Model file for the job. Use its own axes, mm. A direction names the side the tool comes from. Coordinates: 2 decimals unless noted, no trailing zeros. Order: outer loops, then holes, each group sorted by start corner. A loop starts at its lowest first (then second) coordinate and runs counter-clockwise, first axis right, second up. Notation, with made-up numbers: (9, -0.5) -> (40, -0.5) arc R19 ccw to (40, 3.5) -> close; hole circle Ø11 at (64, 75). An arc over 180 degrees is marked (long way). Return JSON: item names as keys, results as strings. Group by question number.
1) Cut at C-C (y = 73.5). Write the cut outline in (x, z).
2) Cut at B-B (z = -26.5). Write the cut outline in (x, y), and give its area (3 significant figures).
3) Probe line 1 (Y direction, x = 41.75, z = -55); line 2 (X direction, y = 2.55, z = 4); line 3 (X direction, y = 2.1, z = -43). List the from-to ranges inside material, lowest first.
4) Cut at A-A (z = -55). State how many separate pieces and enclosed holes the cut face has, and give its area (3 significant figures).
5) Flat gauge pins, fed straight in: pin 1 (8 mm diameter, centred on x = 38.5, y = 87.5, fed in from +Z); pin 2 (4 mm diameter, centred on x = 33, z = -80.5, fed in from -Y); pin 3 (4 mm diameter, centred on y = 28, z = -54.5, fed in from -X). Where does each tip first touch, or does it go through?
6) Which spindle directions (+Z, -Z, +X, -X, +Y, -Y) get a long thin tool onto all of the face, cutting with end or side? Do faces 1 (the cylindrical face through (38.19, 2.96, -41.45)), 2 (the flat face through (38, 126, -30)), 3 (the flat face through (34.97, 41.13, -55.07)), 4 (the flat face through (38, 121, -83)), 5 (the flat face through (38, 71, 22)). Say none if no direction does.
7) Pull direction Y, two halves, no side cores. Call faces 6 (the flat face through (28, 49, 10)), 7 (the flat face through (13.7, 39.5, -5.1)), 8 (the flat face through (6.375, 17.042, -55.07)): +Y half, -Y half, draft (parallel to the pull), parting line (faces both ways), or undercut.
from build123d import *

# Parameters (mm, degrees)
SKETCH_1_W          = 35
SKETCH_1_H          = 60
SKETCH_1_W_2        = 8
EXTRUDE_1_DEPTH     = 6
HOLE_WIZARD_1_D     = 3.5
FILLET_1_R          = 3
SKETCH_5_W          = 10
SKETCH_5_H          = 10
EXTRUDE_2_DEPTH     = 120
SKETCH_10_W         = 10
SKETCH_10_H         = 60
EXTRUDE_5_DEPTH     = 10
HOLE_WIZARD_2_D     = 3.5
HOLE_WIZARD_3_D     = 6
HOLE_WIZARD_3_DEPTH = 4
EXTRUDE_6_DEPTH     = 10
SKETCH_18_W         = 35
SKETCH_18_H         = 15
EXTRUDE_7_DEPTH     = 10
HOLE_WIZARD_4_D     = 4
FILLET_2_R          = 10
FILLET_3_R          = 3
SKETCH_21_W         = 10
SKETCH_21_H         = 10
EXTRUDE_8_DEPTH     = 6
HOLE_WIZARD_5_D     = 4
SKETCH_25_W         = 10
SKETCH_25_H         = 10
EXTRUDE_9_DEPTH     = 10
SKETCH_28_W         = 4
SKETCH_28_H         = 8
CUT_EXTRUDE_1_DEPTH = 172.37677789
CUT_EXTRUDE_2_DEPTH = 172.37677789


with BuildPart() as part:
    # 草图1 → 凸台-拉伸1 (new body)
    with BuildSketch(Plane(origin=(0, 0, 0), x_dir=(1, 0, 0), z_dir=(0, 1, 0))):
        Polygon((18, 68), (18, 60), (35, 60), (43, 60), (43, 68), align=None)
        with Locations((17.5, 30)):
            Rectangle(SKETCH_1_W, SKETCH_1_H)
        with Locations((39, 30)):
            Rectangle(SKETCH_1_W_2, SKETCH_1_H)
        Polygon((35, 0), (18, 0), (18, -8), (43, -8), (43, 0), align=None)
    extrude(amount=EXTRUDE_1_DEPTH)

    # 孔1 (through all)
    with Locations(Plane(origin=(0, 6, 0), x_dir=(1, 0, 0), z_dir=(0, 1, 0))):
        with Locations((24, 64), (39, 43), (39, 17), (24, -4)):
            Hole(HOLE_WIZARD_1_D / 2)

    # 圆角1
    fillet_1_edges = [part.edges().sort_by_distance(p)[0] for p in [
        (18, 3, 8),
        (18, 3, 0),
        (18, 3, -68),
        (43, 3, -68),
        (43, 3, 8),
    ]]
    fillet(fillet_1_edges, radius=FILLET_1_R)

    # 草图5 → 凸台-拉伸2 (add)
    with BuildSketch(Plane(origin=(0, 6, 0), x_dir=(1, 0, 0), z_dir=(0, 1, 0))):
        with Locations((38, 55)):
            Rectangle(SKETCH_5_W, SKETCH_5_H)
        with Locations((38, 5)):
            Rectangle(SKETCH_5_W, SKETCH_5_H)
    extrude(amount=EXTRUDE_2_DEPTH)

    # 草图10 → 凸台-拉伸5 (add)
    with BuildSketch(Plane(origin=(0, 126, 0), x_dir=(1, 0, 0), z_dir=(0, 1, 0))):
        with Locations((38, 30)):
            Rectangle(SKETCH_10_W, SKETCH_10_H)
    extrude(amount=EXTRUDE_5_DEPTH)

    # 孔2 (through all)
    with Locations(Plane(origin=(43, 0, 0), x_dir=(0, 0, -1), z_dir=(1, 0, 0))):
        with Locations((5, 131), (55, 131), (55, 80), (5, 80)):
            Hole(HOLE_WIZARD_2_D / 2)

    # 孔3
    with Locations(Plane(origin=(43, 0, 0), x_dir=(0, 0, -1), z_dir=(1, 0, 0))):
        with Locations((5, 131), (5, 80), (55, 80), (55, 131)):
            Hole(HOLE_WIZARD_3_D / 2, depth=HOLE_WIZARD_3_DEPTH)

    # 草图16 → 凸台-拉伸6 (add)
    with BuildSketch(Plane(origin=(0, 0, -60), x_dir=(-1, 0, 0), z_dir=(0, 0, -1))):
        Polygon((-33, 51.15767665), (-6.92820323, 6), (0, 6), (-33, 63.15767665), align=None)
    extrude_6 = extrude(amount=-EXTRUDE_6_DEPTH)

    # 镜向1: 凸台-拉伸6 across plane
    add(extrude_6.mirror(Plane.XY.offset(-30)))

    # 草图18 → 凸台-拉伸7 (add)
    with BuildSketch(Plane.ZY.offset(-33)):
        with Locations((-77.5, 128.5)):
            Rectangle(SKETCH_18_W, SKETCH_18_H)
        with Locations((17.5, 128.5)):
            Rectangle(SKETCH_18_W, SKETCH_18_H)
        with Locations((-77.5, 63.5)):
            Rectangle(SKETCH_18_W, SKETCH_18_H)
        with Locations((17.5, 63.5)):
            Rectangle(SKETCH_18_W, SKETCH_18_H)
    extrude(amount=-EXTRUDE_7_DEPTH)

    # 孔4 (through all)
    with Locations(Plane.ZY.offset(-33)):
        with Locations((-87.5, 129), (27.5, 129), (27.5, 63), (-87.5, 63)):
            Hole(HOLE_WIZARD_4_D / 2)

    # 圆角2
    fillet_2_edges = [part.edges().sort_by_distance(p)[0] for p in [
        (38, 121, -60),
        (38, 121, 0),
        (38, 71, -60),
        (38, 71, 0),
    ]]
    fillet(fillet_2_edges, radius=FILLET_2_R)

    # 圆角3
    fillet_3_edges = [part.edges().sort_by_distance(p)[0] for p in [
        (18, 3, -60),
    ]]
    fillet(fillet_3_edges, radius=FILLET_3_R)

    # 草图21 → 凸台-拉伸8 (add)
    with BuildSketch(Plane(origin=(-2.598076211, 1.5, 0), x_dir=(0, 0, 1), z_dir=(-0.8660254037844363, 0.5000000000000042, 0))):
        Polygon((-60, 51.059600438), (-70, 51.059600438), (-60, 41.059600438), align=None)
        with Locations((-65, 56.059600438)):
            Rectangle(SKETCH_21_W, SKETCH_21_H)
        with Locations((5, 56.059600438)):
            Rectangle(SKETCH_21_W, SKETCH_21_H)
        Polygon((0, 51.059600438), (10, 51.059600438), (0, 41.059600438), align=None)
    extrude(amount=-EXTRUDE_8_DEPTH)

    # 孔5 (through all)
    with Locations(Plane(origin=(-2.598076211, 1.5, 0), x_dir=(0, 0, 1), z_dir=(-0.8660254037844363, 0.5000000000000042, 0))):
        with Locations((-62, 56.059600438), (2, 56.059600438)):
            Hole(HOLE_WIZARD_5_D / 2)

    # 草图25 → 凸台-拉伸9 (add)
    with BuildSketch(Plane(origin=(-2.598076211, 1.5, 0), x_dir=(0, 0, 1), z_dir=(-0.8660254037844363, 0.5000000000000042, 0))):
        with Locations((-55, 36.059600438)):
            Rectangle(SKETCH_25_W, SKETCH_25_H)
        with Locations((-5, 36.059600438)):
            Rectangle(SKETCH_25_W, SKETCH_25_H)
    extrude(amount=EXTRUDE_9_DEPTH)

    # 草图28 → 切除-拉伸1 (cut, through all)
    with BuildSketch(Plane(origin=(0, 0, -60), x_dir=(-1, 0, 0), z_dir=(0, 0, -1))):
        with Locations((-35, 47.15767665)):
            Rectangle(SKETCH_28_W, SKETCH_28_H)
    extrude(amount=-CUT_EXTRUDE_1_DEPTH, mode=Mode.SUBTRACT)

    # 草图29 → 切除-拉伸2 (cut, through all)
    with BuildSketch(Plane(origin=(0, 0, -60), x_dir=(-1, 0, 0), z_dir=(0, 0, -1))):
        Polygon((-37, 43.15767665), (-33, 43.15767665), (-33, 39.15767665), align=None)
    extrude(amount=-CUT_EXTRUDE_2_DEPTH, mode=Mode.SUBTRACT)


solid = part.part
Answers below:
{
 "1": {"outline": "(33, -63.39) -> (43, -63.39) -> (43, -50) -> (33, -50) -> close; (33, -10) -> (43, -10) -> (43, 3.39) -> (33, 3.39) -> close"},
 "2": {"outline": "(0, 0) -> (43, 0) -> (43, 6) -> (0, 6) -> close; (33, 126) -> (43, 126) -> (43, 136) -> (33, 136) -> close", "area": "358 mm^2"},
 "3": {"line 1": "y = 0 to 77, 83 to 128, 134 to 136", "line 2": "x = 18 to 22.25, 25.75 to 43", "line 3": "x = 0 to 37.25, 40.75 to 43"},
 "4": {"separate pieces": "3", "enclosed holes": "1", "area": "1,880 mm^2"},
 "5": {"pin 1": "stops at z = 0", "pin 2": "stops at y = 56", "pin 3": "stops at x = 10.16"},
 "6": {"face 1": "-Y", "face 2": "+X, -X", "face 3": "+Z, -Z", "face 4": "-Z, +X, -X", "face 5": "+Z, +X, -X"},
 "7": {"face 6": "draft", "face 7": "+Y half", "face 8": "undercut"}
}
